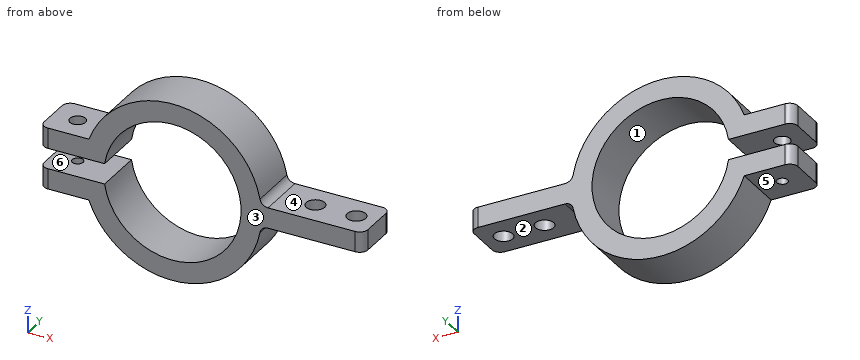
Autodesk Inventor part; units mm, degrees
ref_plane "Work Plane3" through (19.75, 0, 0) normal (1, 0, 0) x (0, 1, 0)
ref_plane "XZ Plane" through (0, 0, 0) normal (0, 1, 0) x (-1, 0, 0)
ref_plane "XY Plane" through (0, 0, 0) normal (0, 0, 1) x (1, 0, 0)
sketch "Sketch1" plane through (0, 0, 0) normal (0, 1, 0) x (-1, 0, 0)
  arc A0 (16.5624, 2.5) -> (16.5624, -2.5) centre (0, 0) ccw
  arc A1 (20.416, 7.5) -> (20.416, -7.5) centre (0, 0) ccw
  line L0 (32.416, 7.5) -> (20.416, 7.5)
  line L1 (16.5624, 2.5) -> (32.416, 2.5)
  line L2 (32.416, 2.5) -> (32.416, 7.5)
  line L3 (32.416, -2.5) -> (16.5624, -2.5)
  line L4 (20.416, -7.5) -> (32.416, -7.5)
  line L5 (32.416, -7.5) -> (32.416, -2.5)
  line L6 (26.416, 5) -> (26.416, -5) construction
  line L7 (-21.6058, -2.5) -> (-46.6058, -2.5)
  line L8 (-46.6058, -2.5) -> (-46.6058, 2.5)
  line L9 (-46.6058, 2.5) -> (-21.6058, 2.5)
  line L10 (-21.6058, 2.5) -> (-21.6058, -2.5)
  point P0 (32.416, 5)
  point P1 (32.416, -5)
  point P2 (26.416, 0)
  point P3 (26.416, -7.5)
  point P4 (-16.75, 0)
  point P5 (-46.6058, 0)
  dimension "d0" = 33.5
  dimension "d1" = 5
  dimension "d4" = 5
  dimension "d5" = 5
  dimension "d6" = 10
  dimension "d7" = 12
  dimension "d35" = 5
  dimension "d36" = 25
extrude "Extrusion1" add sketch "Sketch1" along normal mid plane 12
sketch "Sketch2" plane through (-32.416, 6, 7.5) normal (0, 0, 1) x (1, 0, 0)
  line L0 (0, 0) -> (0, -12)
  line L1 (0, 0) -> (12, 0)
  point P0 (32.416, -6)
  point P1 (6, -6)
  point P2 (0, -6)
  point P3 (6, 0)
hole "Hole1" at (-26.416, 0, 7.5) direction (0, 0, -1) diameter 3.797 depth 5
sketch "Sketch3" plane through (-20.416, 6, -7.5) normal (0, 0, -1) x (-1, 0, 0)
  line L0 (8.3161, -1.9884) -> (10.6322, -6)
  line L1 (10.6322, -6) -> (8.3161, -10.0116)
  line L2 (8.3161, -10.0116) -> (3.6839, -10.0116)
  line L3 (3.6839, -10.0116) -> (1.3678, -6)
  line L4 (1.3678, -6) -> (3.6839, -1.9884)
  line L5 (3.6839, -1.9884) -> (8.3161, -1.9884)
  circle A0 centre (6, -6) radius 1.8985
  point P0 (-20.416, -6)
  dimension "d17" = 8.0232
extrude "Extrusion2" [suppressed]
ref_plane "Work Plane3" through (19.75, 0, 0) normal (1, 0, 0) x (0, 1, 0)
sketch "Sketch6" plane through (-20.416, -6, -7.5) normal (0, 0, -1) x (-1, 0, 0)
  line L0 (12, 0) -> (-3.8536, 0)
  point P0 (-20.416, 6)
  point P1 (10, 0)
  point P2 (6, 6)
hole "Hole3" at (-26.416, 0, -7.5) direction (0, 0, 1) diameter 2.642 depth 5
sketch "Sketch7" plane through (21.6058, 6, 2.5) normal (0, 0, 1) x (1, 0, 0)
  line L0 (25, -12) -> (25, 0)
  point P0 (-21.6058, -6)
  point P1 (20, -6)
  point P2 (10, -6)
  point P3 (25, -6)
  dimension "d44" = 5
  dimension "d45" = 10
hole "Hole4" at (41.6058, 0, 2.5) at (31.6058, 0, 2.5) direction (0, 0, -1) diameter 4.496 end through all
fillet "Fillet2" radius 2 6 edges at (46.6058, -6, 0) (46.6058, 6, 0) (-32.416, -6, 5) (-32.416, 6, 5) (-32.416, 6, -5) (-32.416, -6, -5)
fillet "Fillet3" radius 2 2 edges at (21.6058, 0, -2.5) (21.6058, 0, 2.5)
equation "\"d5\" = d4"
properties part number "CameraClampRotate"
Can you work these out from the model? Positions are in its coordinate system, mm. Face numbers are marked on the shaded views. A direction names the side the tool comes from. Give positions to 0.01 mm unless a question says otherwise; leave off trailing zeros. Write each loop counter-clockwise with the first axis right and the second up, starting at its lowest first coordinate (ties: lowest second). Pieces come first, ordered by that corner, then holes. Notation, with made-up numbers: (-37.5, -35.75) - (-18.5, -35.75) arc R8 cw to (-18.5, -24.75) - close; hole circle Ø10 at (89.25, 27). An arc over 180 degrees is marked (long way). Write item = value, one per line. Start each with the question number.
1. Please list where these lines run through material, in increasing order: line 1 (X direction, y = 0, z = 0.55); line 2 (X direction, y = 0, z = 4); line 3 (Z direction, x = -13, y = 2.5).
2. Imagine slicing it at C-C (z = 10). Please give me the cut outline in (x, y), and give its area (3 significant figures).
3. For pin 1 (5 mm diameter, centred on x = 10.5, y = 0.5, fed in from -Z); pin 2 (5 mm diameter, centred on x = 41.61, y = 0, fed in from +Z); pin 3 (1.5 mm diameter, centred on y = -2.5, z = -17, fed in from +X), each with a flat end and sliding along its axis, tell me the tip position at first contact or that it passes through.
4. Thinking about a two-plate mould opening in Z: for the marked faces 1, 2 and 3, which applies, released by +Z, released by -Z, zero draft, split by the parting line, or undercut?
5. Imagine slicing it at D-D (y = 3.25). Please give me the cut outline in (x, z).
6. Imagine slicing it at B-B (y = 0). Count the separate pieces of the cut face and the enclosed holes in it, and give its area (3 significant figures).
7. Imagine slicing it at A-A (x = 0). Please give me the cut outline in (y, z).
8. On a 3-axis mill with a long thin cutter (end or side, diameter ignored), from which of +Z, -Z, +X, -X, +Y, -Y can I reach the whole of each face in a straight line? I mean the marked faces 4, 5 and 6. Say none if no direction works.
Worked answers:
q1.line_1 = 16.74 to 29.36, 33.85 to 39.36, 43.85 to 46.61
q1.line_2 = -32.42 to -28.31, -24.52 to -16.27, 16.27 to 21.38
q1.line_3 = -17.44 to -10.56, 10.56 to 17.44
q2.outline = (-19.31, -6) - (-13.44, -6) - (-13.44, 6) - (-19.31, 6) - close; (13.44, -6) - (19.31, -6) - (19.31, 6) - (13.44, 6) - close
q2.area = 141 mm2
q3.pin_1 = -20.23
q3.pin_2 = 2.5
q3.pin_3 = 14.46
q4.face_1 = undercut
q4.face_2 = released by -Z
q4.face_3 = zero draft
q5.outline = (-32.42, -7.5) - (-20.42, -7.5) arc R21.75 ccw to (21.36, -4.12) arc R2 cw to (23.32, -2.5) - (46.61, -2.5) - (46.61, 2.5) - (23.32, 2.5) arc R2 cw to (21.36, 4.12) arc R21.75 ccw to (-20.42, 7.5) - (-32.42, 7.5) - (-32.42, 2.5) - (-16.56, 2.5) arc R16.75 cw (long way) to (-16.56, -2.5) - (-32.42, -2.5) - close
q6.separate_pieces = 5
q6.enclosed_holes = 0
q6.area = 741 mm2
q7.outline = (-6, -21.75) - (6, -21.75) - (6, -16.75) - (-6, -16.75) - close; (-6, 16.75) - (6, 16.75) - (6, 21.75) - (-6, 21.75) - close
q8.face_4 = +Z, +X, +Y, -Y
q8.face_5 = -Z, -X, +Y, -Y
q8.face_6 = -X, +Y, -Y
